from build123d import *

# Parameters (mm, degrees)
F1_DEPTH = 9.525


with BuildPart() as f1:
    # F0 (on Top) → F1 (new body)
    with BuildSketch(Plane.XY):
        with BuildLine():
            ThreePointArc((-21.264499, -28.660992), (-36.472978, -26.406095), (-50.372925, -19.835413))
            ThreePointArc((-50.372925, -19.835413), (-37.692308, -32.991899), (-21.264499, -40.993041))
            Line((-21.264499, -40.993041), (-21.264499, -47.747492))
            Line((-21.264499, -47.747492), (7.390787, -47.747492))
            Line((7.390787, -47.747492), (7.390787, -41.019611))
            ThreePointArc((7.390787, -41.019611), (30.151885, -27.661847), (43.512857, -4.902632))
            Line((43.512857, -4.902632), (50.226257, -4.902632))
            Line((50.226257, -4.902632), (50.226257, 23.754346))
            Line((50.226257, 23.754346), (43.489843, 23.754346))
            ThreePointArc((43.489843, 23.754346), (35.483013, 40.193269), (22.314296, 52.879184))
            ThreePointArc((22.314296, 52.879184), (28.893077, 38.972268), (31.150838, 23.754346))
            Line((31.150838, 23.754346), (7.390787, 23.754346))
            Line((7.390787, 23.754346), (7.390787, 66.552508))
            Line((7.390787, 66.552508), (-21.264499, 66.552508))
            Line((-21.264499, 66.552508), (-21.241715, 23.707046))
            Line((-21.241715, 23.707046), (-64.073743, 23.707046))
            Line((-64.073743, 23.707046), (-64.073743, -4.902632))
            Line((-64.073743, -4.902632), (-21.264499, -4.902632))
            Line((-21.264499, -4.902632), (-21.264499, -28.660992))
        make_face()
        with BuildLine():
            Line((7.390787, -20.13463), (7.390787, -4.902632))
            Line((7.390787, -4.902632), (22.623372, -4.902632))
            ThreePointArc((22.623372, -4.902632), (15.798027, -13.309609), (7.390787, -20.13463))
        make_face(mode=Mode.SUBTRACT)
    extrude(amount=F1_DEPTH)


solid = f1.part
Design review of the part built by this model. Coordinates are the model's own, in mm. A direction names the side the tool comes from. Round coordinates to 2 decimals unless told otherwise and drop trailing zeros. Write each loop counter-clockwise with the first axis right and the second up, starting at its lowest first coordinate (ties: lowest second). Pieces come first, ordered by that corner, then holes. Notation, with made-up numbers: M -9,40.5 L 3,40.5 A16 ccw 3,49.5 Z; hole C -40,29 d7. An arc over 180 degrees is marked long. One line per item, written item: value. Start each with the question number.
1. Clearance check with flat-ended pins moving along their axes: P1, Ø5, axis at x = 18.5, z = 3.5, coming from the -Y side; P2, Ø3.5, axis at y = -44, z = 3.5, coming from the +X side; P3, Ø2, axis at x = -2, y = 8, coming from the -Z side; P4, Ø2, axis at y = -30, z = 6.5, coming from the +X side. State where each tip first meets the part, or that it passes through.
2. Take a section at A-A on z = 4.5. State the section outline as (x, y) points, then the cut area to 3 significant figures.
3. For faces 5 (the face through (47, 23.754, 5)), 6 (the face through (-36.266, -26.468, 4.696)), 7 (the face through (7.391, 45, 5)), list the 3-axis set-ups (+Z, -Z, +X, -X, +Y, -Y) from which the entire face can be reached by the end or side of a thin tool; tool diameter is ignored.
4. Take a section at C-C on y = 42. State the section outline as (x, z) points (3 decimals), then the cut area to 3 significant figures.
5. Draft analysis for pull direction X (two halves, no side actions). For faces 1 (the face through (-64.074, 10, 5)), 2 (the face through (15.91, -13.2, 4.7)), 3 (the face through (29.89, -27.92, 4.7)), 4 (the face through (28.83, 39.18, 4.7)), state which applies: pulls with the +X half, pulls with the -X half, needs draft (parallel to the pull), parting line crosses it, or undercut.
6. Take a section at D-D on x = -57. State the section outline as (y, z) points (3 decimals), then the cut area to 3 significant figures.
7. Take a section at B-B on x = 27. State the section outline as (y, z) points (3 decimals).
8. To check wall thickness, follow probe 1 along Y at (x, z) = (-22, 5); probe 2 along Y at (x, z) = (-34, 3.5); probe 3 along X at (y, z) = (-22, 8). State the ranges of each line that lie inside material, in increasing order. Write a range as from..to.
Computed:
1. P1: stops at y = -37.74
1. P2: stops at x = 7.39
1. P3: stops at z = 0
1. P4: stops at x = 28.76
2. outline: M -64.07,-4.9 L -21.26,-4.9 L -21.26,-28.66 A52.42 cw -50.37,-19.84 A52.39 ccw -21.26,-40.99 L -21.26,-47.75 L 7.39,-47.75 L 7.39,-41.02 A52.39 ccw 43.51,-4.9 L 50.23,-4.9 L 50.23,23.75 L 43.49,23.75 A52.39 ccw 22.31,52.88 A52.42 cw 31.15,23.75 L 7.39,23.75 L 7.39,66.55 L -21.26,66.55 L -21.24,23.71 L -64.07,23.71 Z; hole M 7.39,-20.13 A52.42 ccw 22.62,-4.9 L 7.39,-4.9 Z
2. area: 6,900 mm²
3. face 5: +Z, -Z, +X, +Y
3. face 6: +Z, -Z
3. face 7: +Z, -Z, +Y
4. outline: M -21.251,0 L 7.391,0 L 7.391,9.525 L -21.251,9.525 Z; M 27.873,0 L 34.109,0 L 34.109,9.525 L 27.873,9.525 Z
4. area: 332 mm²
5. face 1: pulls with the -X half
5. face 2: undercut
5. face 3: pulls with the +X half
5. face 4: undercut
6. outline: M -4.903,0 L 23.707,0 L 23.707,9.525 L -4.903,9.525 Z
6. area: 273 mm²
7. outline: M -30.565,0 L 23.754,0 L 23.754,9.525 L -30.565,9.525 Z; M 44.197,0 L 49.336,0 L 49.336,9.525 L 44.197,9.525 Z
8. probe 1: y = -40.78..-28.66, -4.9..23.71
8. probe 2: y = -35.44..-27.09, -4.9..23.71
8. probe 3: x = -48.84..-46.84, -21.26..35.06
